from build123d import *

# Parameters (mm, degrees)
F0_R     = 3.048
F1_DEPTH = 4.7625
F2_R     = 4.7625
F3_DEPTH = 9.525
F4_R     = 2.54
F4_R_2   = 1.4605
F5_DEPTH = 0.79375


# Not quite as in the source:
# - a length typed as a fraction of an inch, garbled in the dataset ("3 / 203.2 mm" for 3/8 in), is restored


with BuildPart() as f1:
    # F0 (on Top) → F1 (new body, symmetric)
    with BuildSketch(Plane.XY):
        Circle(F0_R)
    extrude(amount=F1_DEPTH, both=True)

    # F2 (on face) → F3 (join)
    with BuildSketch(Plane.XY.offset(4.7625)):
        Circle(F2_R)
    extrude(amount=F3_DEPTH)

    # F4 (on face) → F5 (cut)
    with BuildSketch(Plane.XY.offset(14.2875)):
        Circle(F4_R)
        Circle(F4_R_2, mode=Mode.SUBTRACT)
    extrude(amount=-F5_DEPTH, mode=Mode.SUBTRACT)


solid = f1.part
Check sheet for the modelled part. Datum: model origin and axes. Units: mm. A direction names the side the tool comes from. Coordinates: 2 decimals unless noted, no trailing zeros. Loops run counter-clockwise (first coordinate to the right, second up) from the corner with the lowest first, then second, coordinate; pieces in that order, holes last. Notation, with made-up numbers: (-11, 25.5) -> (31, 25.5) arc R16 cw to (31, 31.5) -> close; hole circle Ø3 at (1.5, 52.5). An arc over 180 degrees is marked (long way). Answer in a Markdown table with one row per item.
1. Access from +Z, -Z, +X, -X, +Y, -Y to the whole of each face (thin tool, end or side, straight path). Record for faces 4 (the face through (1, -3.1, 4.762)), 5 (the face through (2, -2, 14.288)), 6 (the face through (-0.33, 2.52, 13.9)).
Check values:
| item | result |
|---|---|
| face 4 | -Z |
| face 5 | +Z, +X, -X, +Y, -Y |
| face 6 | +Z |
2. Sectioned sample at C-C, the plane z = 2.25. Record the boundary of the cut face in (x, y), then the cut area to 3 significant figures.
Check values:
| item | result |
|---|---|
| outline | circle Ø6.1 at (0, 0) |
| area | 29.2 mm2 |
3. Material ranges on line 1 along Y through (x, z) = (0, 14); line 2 along Z through (x, y) = (-3.75, 1); line 3 along Z through (x, y) = (0.25, 1.5), recorded low to high. Write a range as [from, to].
Check values:
| item | result |
|---|---|
| line 1 | y = [-4.76, -2.54], [-1.46, 1.46], [2.54, 4.76] |
| line 2 | z = [4.76, 14.29] |
| line 3 | z = [-4.76, 13.49] |
4. Sectioned sample at D-D, the plane y = -2. Record the boundary of the cut face in (x, z), then the cut area to 3 significant figures.
Check values:
| item | result |
|---|---|
| outline | (-4.32, 4.76) -> (-2.3, 4.76) -> (-2.3, -4.76) -> (2.3, -4.76) -> (2.3, 4.76) -> (4.32, 4.76) -> (4.32, 14.29) -> (1.57, 14.29) -> (1.57, 13.49) -> (-1.57, 13.49) -> (-1.57, 14.29) -> (-4.32, 14.29) -> close |
| area | 124 mm2 |
5. Sectioned sample at A-A, the plane x = 0. Record the boundary of the cut face in (y, z).
Check values:
| item | result |
|---|---|
| outline | (-4.76, 4.76) -> (-3.05, 4.76) -> (-3.05, -4.76) -> (3.05, -4.76) -> (3.05, 4.76) -> (4.76, 4.76) -> (4.76, 14.29) -> (2.54, 14.29) -> (2.54, 13.49) -> (1.46, 13.49) -> (1.46, 14.29) -> (-1.46, 14.29) -> (-1.46, 13.49) -> (-2.54, 13.49) -> (-2.54, 14.29) -> (-4.76, 14.29) -> close |
6. Go/stop test with flat-tipped pins: pin 1 (1 mm diameter, centred on y = -0.5, z = 6, fed in from +X); pin 2 (3 mm diameter, centred on y = -2.5, z = -2, fed in from +X); pin 3 (5 mm diameter, centred on x = 0.5, z = -2.5, fed in from -Y); pin 4 (3 mm diameter, centred on x = -2.5, z = 10, fed in from -Y). Record where each tip stops, or that it passes through.
Check values:
| item | result |
|---|---|
| pin 1 | stops at x = 4.76 |
| pin 2 | stops at x = 2.88 |
| pin 3 | stops at y = -3.05 |
| pin 4 | stops at y = -4.66 |
7. Release check for a two-part mould opening along X. For faces 1 (the face through (-0.317, -1.426, 13.896)), 2 (the face through (-0.4, 3.02, 0.07)), 3 (the face through (0, 0, 14.288)) record: released by +X, released by -X, zero draft, split by the parting line, or undercut.
Check values:
| item | result |
|---|---|
| face 1 | undercut |
| face 2 | split by the parting line |
| face 3 | zero draft |
